```python
from build123d import *

# Parameters (mm, degrees)
EXTRUDE_1_DEPTH               = 65
SKETCH_4_W                    = 112
SKETCH_4_H                    = 50
CUT_EXTRUDE_1_DEPTH           = 20
SKETCH_5_W                    = 130
SKETCH_5_H                    = 50
SKETCH_5_R                    = 6.55
SKETCH_5_R_2                  = 1.5
EXTRUDE_2_DEPTH               = 3
SKETCH_6_R                    = 1.2
CUT_EXTRUDE_2_DEPTH           = 20
SKETCH_7_R                    = 1.5
CUT_EXTRUDE_3_DEPTH           = 20
SKETCH_8_R                    = 2.65
CUT_EXTRUDE_4_DEPTH           = 2
CUT_EXTRUDE_4_DRAFT           = -25
CUT_EXTRUDE_4_PROFILE_2_DEPTH = 2
CUT_EXTRUDE_4_PROFILE_2_DRAFT = -25
CUT_EXTRUDE_4_PROFILE_3_DEPTH = 2
CUT_EXTRUDE_4_PROFILE_3_DRAFT = -25
CUT_EXTRUDE_4_PROFILE_4_DEPTH = 2
CUT_EXTRUDE_4_PROFILE_4_DRAFT = -25
CUT_EXTRUDE_5_DEPTH           = 5


with BuildPart() as part:
    # Sketch 2 → Extrude 1 (new, symmetric)
    with BuildSketch(Plane(origin=(0, 0, 0), x_dir=(0, 0, -1), z_dir=(1, 0, 0))):
        with BuildLine():
            Line((-7.45, 12), (7.45, 12))
            ThreePointArc((7.45, 12), (10, 9.45), (12.55, 12))
            Line((12.55, 12), (32, 12))
            Line((32, 12), (32, 0))
            Line((32, 0), (-18, 0))
            Line((-18, 0), (-18, 12))
            Line((-18, 12), (-12.55, 12))
            ThreePointArc((-12.55, 12), (-10, 9.45), (-7.45, 12))
        make_face()
    extrude(amount=EXTRUDE_1_DEPTH, both=True)

    # Sketch 4 → Cut-Extrude 1 (cut)
    with BuildSketch(Plane.XZ):
        with Locations((0, -7)):
            Rectangle(SKETCH_4_W, SKETCH_4_H)
    extrude(amount=-CUT_EXTRUDE_1_DEPTH, mode=Mode.SUBTRACT)


with BuildPart() as cut_extrude_1_piece_1:
    # of the separate pieces the step leaves, piece 1, a body of its own (cut_extrude_1_pieces)
    add(part.part.solids().sort_by_distance((-65, 12, 7.45))[0])



with BuildPart() as cut_extrude_1_piece_2:
    # of the separate pieces the step leaves, piece 2, a body of its own (cut_extrude_1_pieces)
    add(part.part.solids().sort_by_distance((56, 12, 7.45))[0])


with BuildPart() as cut_extrude_1_piece_1_1:
    add(cut_extrude_1_piece_1.part)

    add(cut_extrude_1_piece_2.part)  # Extrude 2 merges Cut-Extrude 1 piece 2
    # Sketch 5 → Extrude 2 (add)
    with BuildSketch(Plane.XZ):
        with Locations((0, -7)):
            Rectangle(SKETCH_5_W, SKETCH_5_H)
        with Locations(Location((0, 0, 0), (0, 0, 270))):
            Circle(SKETCH_5_R, mode=Mode.SUBTRACT)
        with Locations(Location((-14.3, 4.95, 0), (0, 0, 270))):
            Circle(SKETCH_5_R_2, mode=Mode.SUBTRACT)
        with Locations(Location((34.3, -4.95, 0), (0, 0, 90))):
            Circle(SKETCH_5_R_2, mode=Mode.SUBTRACT)
        with Locations(Location((34.3, 4.95, 0), (0, 0, 270))):
            Circle(SKETCH_5_R_2, mode=Mode.SUBTRACT)
        with Locations(Location((-14.3, -4.95, 0), (0, 0, 90))):
            Circle(SKETCH_5_R_2, mode=Mode.SUBTRACT)
        with Locations(Location((-34.3, 4.95, 0), (0, 0, 90))):
            Circle(SKETCH_5_R_2, mode=Mode.SUBTRACT)
        with Locations(Location((-34.3, -4.95, 0), (0, 0, 270))):
            Circle(SKETCH_5_R_2, mode=Mode.SUBTRACT)
        with Locations(Location((14.3, -4.95, 0), (0, 0, 270))):
            Circle(SKETCH_5_R_2, mode=Mode.SUBTRACT)
        with Locations(Location((14.3, 4.95, 0), (0, 0, 90))):
            Circle(SKETCH_5_R_2, mode=Mode.SUBTRACT)
    extrude(amount=EXTRUDE_2_DEPTH)

    # Sketch 6 → Cut-Extrude 2 (cut)
    with BuildSketch(Plane(origin=(0, 12, 0), x_dir=(1, 0, 0), z_dir=(0, 1, 0))):
        with Locations(Location((-60.5, -15.275, 0), (0, 0, 270))):
            Circle(SKETCH_6_R)
        with Locations(Location((-60.5, -4.725, 0), (0, 0, 90))):
            Circle(SKETCH_6_R)
        with Locations(Location((-60.5, 15.275, 0), (0, 0, 90))):
            Circle(SKETCH_6_R)
        with Locations(Location((-60.5, 4.725, 0), (0, 0, 270))):
            Circle(SKETCH_6_R)
        with Locations(Location((-60.5, 29.275, 0), (0, 0, 270))):
            Circle(SKETCH_6_R)
        with Locations(Location((60.5, 29.275, 0), (0, 0, 90))):
            Circle(SKETCH_6_R)
        with Locations(Location((60.5, 4.725, 0), (0, 0, 90))):
            Circle(SKETCH_6_R)
        with Locations(Location((60.5, 15.275, 0), (0, 0, 270))):
            Circle(SKETCH_6_R)
        with Locations(Location((60.5, -4.725, 0), (0, 0, 270))):
            Circle(SKETCH_6_R)
        with Locations(Location((60.5, -15.275, 0), (0, 0, 90))):
            Circle(SKETCH_6_R)
    extrude(amount=-CUT_EXTRUDE_2_DEPTH, mode=Mode.SUBTRACT)

    # Sketch 7 → Cut-Extrude 3 (cut)
    with BuildSketch(Plane.XZ.offset(3)):
        with Locations(Location((-15, -28, 0), (0, 0, 270))):
            Circle(SKETCH_7_R)
        with Locations(Location((-45, -28, 0), (0, 0, 270))):
            Circle(SKETCH_7_R)
        with Locations(Location((45, -28, 0), (0, 0, 270))):
            Circle(SKETCH_7_R)
        with Locations(Location((15, -28, 0), (0, 0, 270))):
            Circle(SKETCH_7_R)
    extrude(amount=-CUT_EXTRUDE_3_DEPTH, mode=Mode.SUBTRACT)


with BuildPart() as cut_extrude_4_tool:
    # Sketch 8 → Cut-Extrude 4 (with draft: the straight prism first)
    with BuildSketch(Plane.XZ.offset(3)):
        with Locations((-45, -28)):
            Circle(SKETCH_8_R)
    extrude(amount=-CUT_EXTRUDE_4_DEPTH)
    # Cut-Extrude 4: the draft: its side faces are tilted about the plane it starts from
    cut_extrude_4_sides = [cut_extrude_4_tool.faces().sort_by_distance(p)[0] for p in [
        (-47.65, -2, -28),
    ]]
    draft(cut_extrude_4_sides, Plane.XZ.offset(3), CUT_EXTRUDE_4_DRAFT)


with BuildPart() as cut_extrude_1_piece_1_2:
    add(cut_extrude_1_piece_1_1.part)

    # Cut-Extrude 4: cut by cut_extrude_4_tool
    add(cut_extrude_4_tool.part, mode=Mode.SUBTRACT)


with BuildPart() as cut_extrude_4_profile_2_tool:
    # Sketch 8 → Cut-Extrude 4 profile 2 (with draft: the straight prism first)
    with BuildSketch(Plane.XZ.offset(3)):
        with Locations((-15, -28)):
            Circle(SKETCH_8_R)
    extrude(amount=-CUT_EXTRUDE_4_PROFILE_2_DEPTH)
    # Cut-Extrude 4 profile 2: the draft: its side faces are tilted about the plane it starts from
    cut_extrude_4_profile_2_sides = [cut_extrude_4_profile_2_tool.faces().sort_by_distance(p)[0] for p in [
        (-17.65, -2, -28),
    ]]
    draft(cut_extrude_4_profile_2_sides, Plane.XZ.offset(3), CUT_EXTRUDE_4_PROFILE_2_DRAFT)


with BuildPart() as cut_extrude_1_piece_1_3:
    add(cut_extrude_1_piece_1_2.part)

    # Cut-Extrude 4 profile 2: cut by cut_extrude_4_profile_2_tool
    add(cut_extrude_4_profile_2_tool.part, mode=Mode.SUBTRACT)


with BuildPart() as cut_extrude_4_profile_3_tool:
    # Sketch 8 → Cut-Extrude 4 profile 3 (with draft: the straight prism first)
    with BuildSketch(Plane.XZ.offset(3)):
        with Locations((15, -28)):
            Circle(SKETCH_8_R)
    extrude(amount=-CUT_EXTRUDE_4_PROFILE_3_DEPTH)
    # Cut-Extrude 4 profile 3: the draft: its side faces are tilted about the plane it starts from
    cut_extrude_4_profile_3_sides = [cut_extrude_4_profile_3_tool.faces().sort_by_distance(p)[0] for p in [
        (12.35, -2, -28),
    ]]
    draft(cut_extrude_4_profile_3_sides, Plane.XZ.offset(3), CUT_EXTRUDE_4_PROFILE_3_DRAFT)


with BuildPart() as cut_extrude_1_piece_1_4:
    add(cut_extrude_1_piece_1_3.part)

    # Cut-Extrude 4 profile 3: cut by cut_extrude_4_profile_3_tool
    add(cut_extrude_4_profile_3_tool.part, mode=Mode.SUBTRACT)


with BuildPart() as cut_extrude_4_profile_4_tool:
    # Sketch 8 → Cut-Extrude 4 profile 4 (with draft: the straight prism first)
    with BuildSketch(Plane.XZ.offset(3)):
        with Locations((45, -28)):
            Circle(SKETCH_8_R)
    extrude(amount=-CUT_EXTRUDE_4_PROFILE_4_DEPTH)
    # Cut-Extrude 4 profile 4: the draft: its side faces are tilted about the plane it starts from
    cut_extrude_4_profile_4_sides = [cut_extrude_4_profile_4_tool.faces().sort_by_distance(p)[0] for p in [
        (42.35, -2, -28),
    ]]
    draft(cut_extrude_4_profile_4_sides, Plane.XZ.offset(3), CUT_EXTRUDE_4_PROFILE_4_DRAFT)


with BuildPart() as cut_extrude_1_piece_1_5:
    add(cut_extrude_1_piece_1_4.part)

    # Cut-Extrude 4 profile 4: cut by cut_extrude_4_profile_4_tool
    add(cut_extrude_4_profile_4_tool.part, mode=Mode.SUBTRACT)

    # Sketch 9 → Cut-Extrude 5 (cut)
    with BuildSketch(Plane.XZ.offset(3)):
        Polygon((-58, -3.281624327), (-60.5, -1.838248654), (-63, -3.281624327), (-63, -6.168375673), (-60.5, -7.611751346), (-58, -6.168375673), align=None)
        Polygon((-58, -13.831624327), (-60.5, -12.388248654), (-63, -13.831624327), (-63, -16.718375673), (-60.5, -18.161751346), (-58, -16.718375673), align=None)
        Polygon((-58, -27.831624327), (-60.5, -26.388248654), (-63, -27.831624327), (-63, -30.718375673), (-60.5, -32.161751346), (-58, -30.718375673), align=None)
        Polygon((-58, 6.168375673), (-60.5, 7.611751346), (-63, 6.168375673), (-63, 3.281624327), (-60.5, 1.838248654), (-58, 3.281624327), align=None)
        Polygon((-58, 13.831624327), (-58, 16.718375673), (-60.5, 18.161751346), (-63, 16.718375673), (-63, 13.831624327), (-60.5, 12.388248654), align=None)
        Polygon((60.5, 12.388248654), (58, 13.831624327), (58, 16.718375673), (60.5, 18.161751346), (63, 16.718375673), (63, 13.831624327), align=None)
        Polygon((58, 3.281624327), (58, 6.168375673), (60.5, 7.611751346), (63, 6.168375673), (63, 3.281624327), (60.5, 1.838248654), align=None)
        Polygon((58, -30.718375673), (58, -27.831624327), (60.5, -26.388248654), (63, -27.831624327), (63, -30.718375673), (60.5, -32.161751346), align=None)
        Polygon((58, -16.718375673), (58, -13.831624327), (60.5, -12.388248654), (63, -13.831624327), (63, -16.718375673), (60.5, -18.161751346), align=None)
        Polygon((58, -6.168375673), (58, -3.281624327), (60.5, -1.838248654), (63, -3.281624327), (63, -6.168375673), (60.5, -7.611751346), align=None)
    extrude(amount=-CUT_EXTRUDE_5_DEPTH, mode=Mode.SUBTRACT)


solid = cut_extrude_1_piece_1_5.part
```
The model under review builds one solid part; all positions refer to its coordinate system, in mm. A direction names the side the tool comes from. Round coordinates to 2 decimals unless told otherwise and drop trailing zeros. Loops run counter-clockwise (first coordinate to the right, second up) from the corner with the lowest first, then second, coordinate; pieces in that order, holes last. Notation, with made-up numbers: (58.25, -11.75) -> (71.25, -11.75) arc R16 cw to (71.25, -0.75) -> close; hole circle Ø5 at (42, 19.5). An arc over 180 degrees is marked (long way). Answer as a JSON object with one key per item and string values. Group by question number.
1) We need section C-C on z = 0. Write out the cut boundary in (x, y), then the cut area to 3 significant figures.
2) For faces 1 (the face through (35.31, -1.48, 6.06)), 2 (the face through (-59.23, -0.54, -27.12)), list the 3-axis set-ups (+Z, -Z, +X, -X, +Y, -Y) from which the entire face can be reached by the end or side of a thin tool; tool diameter is ignored.
3) We need section A-A on x = 45. Write out the cut boundary in (y, z).
4) We need section B-B on y = 6. Give the number of separate pieces and of enclosed holes in the cut face, then the cut area to 3 significant figures.
5) We need section D-D on x = 0. Write out the cut boundary in (y, z), then the cut area to 3 significant figures.
6) For line 1 (X direction, y = -1.5, z = 14); line 2 (X direction, y = 10, z = -15.5); line 3 (X direction, y = 6.25, z = -28), list the stretches that pass through material, from the lowest coordinate up. Write a range as [from, to].
7) For pin 1 Ø3 at (x, z) = (60.5, -15.275) entering from -Y; pin 2 Ø4 at (x, z) = (-25, -3) entering from +Y, all flat-tipped, find the tip position at first contact; note any pin that passes through.
Result set:
{
 "1": {"outline": "(-65, -3) -> (-6.55, -3) -> (-6.55, 0) -> (-56, 0) -> (-56, 12) -> (-65, 12) -> close; (6.55, -3) -> (65, -3) -> (65, 12) -> (56, 12) -> (56, 0) -> (6.55, 0) -> close", "area": "567 mm²"},
 "2": {"face 1": "+Y, -Y", "face 2": "-Y"},
 "3": {"outline": "(-3, -32) -> (0, -32) -> (0, -29.5) -> (-1, -29.5) -> (-1, -29.72) -> (-3, -30.65) -> close; (-3, -25.35) -> (-1, -26.28) -> (-1, -26.5) -> (0, -26.5) -> (0, 18) -> (-3, 18) -> close"},
 "4": {"separate pieces": "2", "enclosed holes": "10", "area": "855 mm²"},
 "5": {"outline": "(-3, -32) -> (0, -32) -> (0, -6.55) -> (-3, -6.55) -> close; (-3, 6.55) -> (0, 6.55) -> (0, 18) -> (-3, 18) -> close", "area": "111 mm²"},
 "6": {"line 1": "[-65, -63], [-58, 58], [63, 65]", "line 2": "[-65, -61.68], [-59.32, -56], [56, 59.32], [61.68, 65]", "line 3": "[-65, -56], [56, 65]"},
 "7": {"pin 1": "y = 2", "pin 2": "y = 0"}
}
